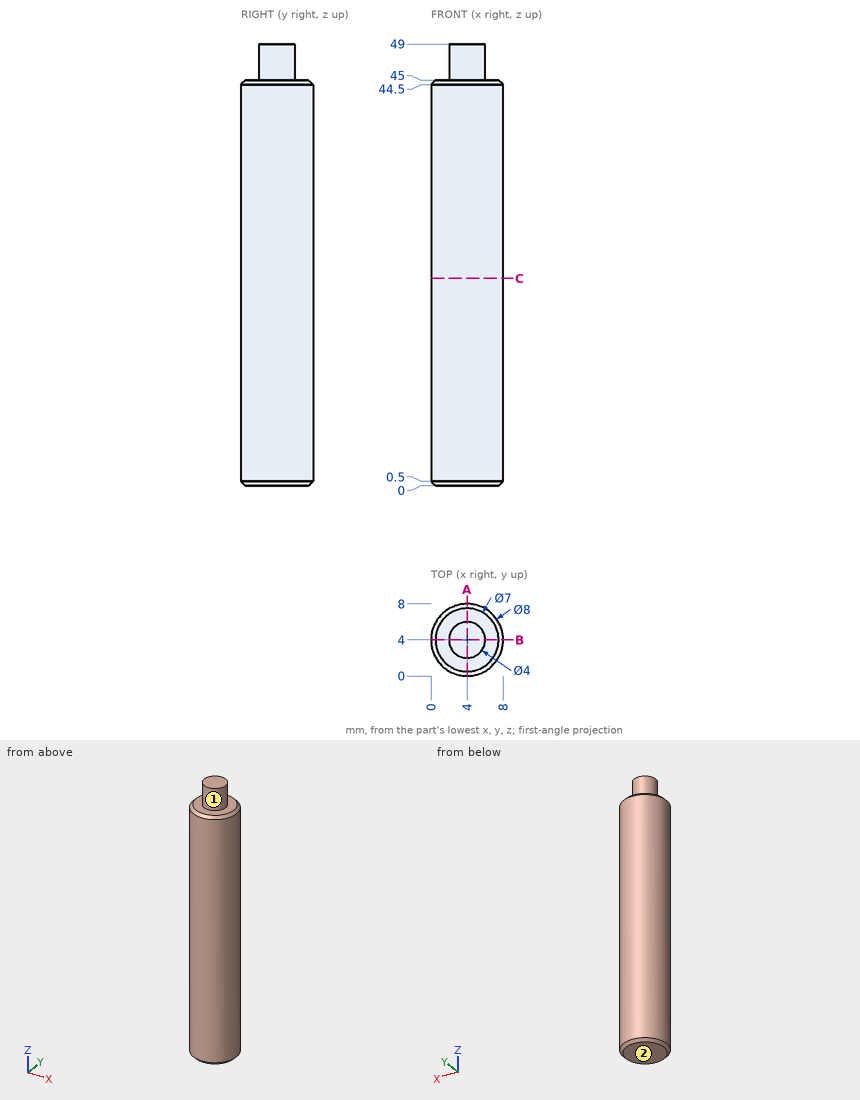
Verification items for this drawing (mm, ordinates from the low corner). A direction names the side the tool comes from. Give positions to 0.01 mm unless a question says otherwise; leave off trailing zeros. Write each loop counter-clockwise with the first axis right and the second up, starting at its lowest first coordinate (ties: lowest second). Pieces come first, ordered by that corner, then holes.
1) Gauge pin test, flat ends, axial feed: pin 1 (4 mm diameter, centred on x = 6, z = 7.5, fed in from -Y); pin 2 (1.5 mm diameter, centred on y = 6.5, z = 26.5, fed in from +X); pin 3 (3 mm diameter, centred on y = 7, z = 40.5, fed in from +X). Record the tip position at first contact, or that the pin passes through.
2) Access from +Z, -Z, +X, -X, +Y, -Y to the whole of each face (thin tool, end or side, straight path). Record for the marked faces 1 and 2.
3) Section check C-C, the plane z = 23. Record the boundary of the cut face in (x, y).
4) Material ranges on L1, parallel to Z at x = 3.75, y = 6.5; L2, parallel to X at y = 4.25, z = 20.5; L3, parallel to Y at x = 3.25, z = 16, recorded low to high.
5) Section check A-A, the plane x = 4. Record the boundary of the cut face in (y, z), and give its area (4 significant figures).
Computed:
1. pin 1: stops at y = 0
1. pin 2: stops at x = 7.6
1. pin 3: stops at x = 7.71
2. face 1: +Z
2. face 2: -Z, +X, -X, +Y, -Y
3. outline: circle Ø8 at (4, 4)
4. L1: z = 0 to 45
4. L2: x = 0.01 to 7.99
4. L3: y = 0.07 to 7.93
5. outline: (0, 0.5) - (0.5, 0) - (7.5, 0) - (8, 0.5) - (8, 44.5) - (7.5, 45) - (6, 45) - (6, 49) - (2, 49) - (2, 45) - (0.5, 45) - (0, 44.5) - close
5. area: 375.5 mm2
